Could you check a few things on this model? Use its own coordinates, in mm. Face numbers are marked on the shaded views. Give positions to 0.01 mm unless a question says otherwise; leave off trailing zeros. Loops run counter-clockwise (first coordinate to the right, second up) from the corner with the lowest first, then second, coordinate; pieces in that order, holes last. Notation, with made-up numbers: (-5, 5) -> (-1, 5) arc R21 ccw to (-1, 23) -> close; hole circle Ø2 at (13, 65). An arc over 180 degrees is marked (long way). Write item = value, one per line. Start each with the question number.
1) I want a section at A-A (x = -10). List the corners of the cut face in (y, z) for me.
2) I'm going to push flat-ended pins straight in: pin 1 Ø3.5 at (x, z) = (10, 0) entering from +Y; pin 2 Ø3 at (y, z) = (1, -2) entering from +X. Where does each tip first touch, or does it pass through?
3) I want a section at D-D (z = 0.5). List the corners of the cut face in (x, y) for me.
4) I want a section at B-B (y = 0.25). Count the separate pieces of the cut face and the enclosed holes in it, and give its area (3 significant figures).
5) If we mould it in two halves opening along X, with no side actions, what happens to the marked faces 1, 2, 3 and 4? For each: +X half, -X half, draft (parallel to the pull), parting line (faces both ways), or undercut.
6) I need wall thicknesses on probe 1 along X at (y, z) = (0, 0); probe 2 along Z at (x, y) = (10, 0); probe 3 along X at (y, z) = (3, -0.5). Which ranges of each line are inside material? Lowest first, please. Write a range as from..to.
7) I want a section at C-C (z = -1.5). List the corners of the cut face in (x, y) for me, and give its area (3 significant figures).
from build123d import *

# Parameters (mm, degrees)
ESBO_O1_W                = 38
ESBO_O1_H                = 8
ESBO_O1_R                = 2
RESSALTO_EXTRUS_O1_DEPTH = 3.25
FILETE1_R                = 4


with BuildPart() as part:
    # Esboço1 → Ressalto-extrusão1 (new, symmetric)
    with BuildSketch(Plane(origin=(0, 0, 0), x_dir=(1, 0, 0), z_dir=(0, 1, 0))):
        Rectangle(ESBO_O1_W, ESBO_O1_H)
        with Locations(Location((-10, 0, 0), (0, 0, 90))):
            Circle(ESBO_O1_R, mode=Mode.SUBTRACT)
        with Locations(Location((10, 0, 0), (0, 0, 90))):
            Circle(ESBO_O1_R, mode=Mode.SUBTRACT)
    extrude(amount=RESSALTO_EXTRUS_O1_DEPTH, both=True)

    # Filete1
    filete1_edges = [part.edges().sort_by_distance(p)[0] for p in [
        (-19, 0, 4),
        (-19, 0, -4),
        (19, 0, -4),
        (19, 0, 4),
    ]]
    fillet(filete1_edges, radius=FILETE1_R - 0.0001)  # a hair under: the kernel refuses the full size


solid = part.part
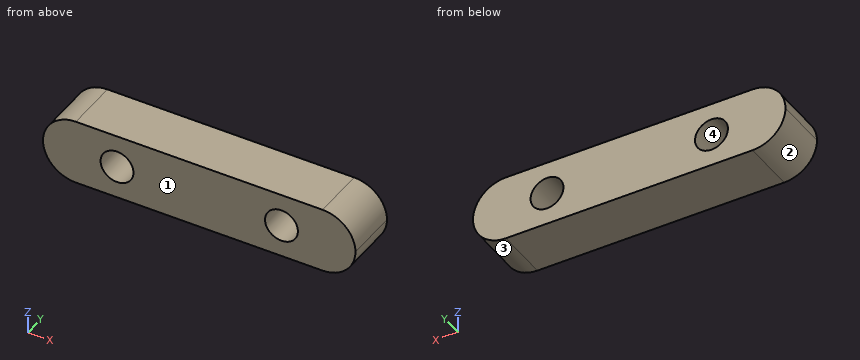
Answer list:
q1.outline = (-3.25, -4) -> (3.25, -4) -> (3.25, -2) -> (-3.25, -2) -> close; (-3.25, 2) -> (3.25, 2) -> (3.25, 4) -> (-3.25, 4) -> close
q2.pin_1 = through
q2.pin_2 = 18.97
q3.outline = (-18.97, -3.25) -> (-11.94, -3.25) -> (-11.94, 3.25) -> (-18.97, 3.25) -> close; (-8.06, -3.25) -> (8.06, -3.25) -> (8.06, 3.25) -> (-8.06, 3.25) -> close; (11.94, -3.25) -> (18.97, -3.25) -> (18.97, 3.25) -> (11.94, 3.25) -> close
q4.separate_pieces = 1
q4.enclosed_holes = 2
q4.area = 265 mm^2
q5.face_1 = draft
q5.face_2 = -X half
q5.face_3 = +X half
q5.face_4 = undercut
q6.probe_1 = -19..-12, -8..8, 12..19
q6.probe_2 = -4..-2, 2..4
q6.probe_3 = -18.97..-11.94, -8.06..8.06, 11.94..18.97
q7.outline = (-18.71, -3.25) -> (-11.32, -3.25) -> (-11.32, 3.25) -> (-18.71, 3.25) -> close; (-8.68, -3.25) -> (8.68, -3.25) -> (8.68, 3.25) -> (-8.68, 3.25) -> close; (11.32, -3.25) -> (18.71, -3.25) -> (18.71, 3.25) -> (11.32, 3.25) -> close
q7.area = 209 mm^2
